```python
from build123d import *

# Parameters (mm, degrees)
F2_DEPTH = 12.5
F3_R     = 1


with BuildPart() as f1:
    # F0 (on Top) → F1 (revolve)
    with BuildSketch(Plane.XY):
        Polygon((-48.5449684441, 34.0502707809), (-50.5449684441, 34.0502707809), (-50.5449684441, 30.5502707809), (-42.7490452468, 30.5502707809), (-42.7490452468, 31.0099636614), (-39.1449684441, 31.2220901251), (-39.1449684441, 32.0502707809), (-41.1449684441, 32.7502707809), (-41.1449684441, 32.4502707809), (-48.5449684441, 32.4502707809), align=None)
        Polygon((-42.7490452468, 31.0099636614), (-42.7490452468, 30.5502707809), (-39.1449684441, 30.5502707809), (-39.1449684441, 31.2220901251), align=None)
    revolve(axis=Axis((-41.4569408685, 30.5502707809, 0), (1, 0, 0)))

    # F0 (on Top) → F2 (cut, symmetric)
    with BuildSketch(Plane.XY):
        Polygon((-42.7490452468, 31.0099636614), (-42.7490452468, 30.5502707809), (-39.1449684441, 30.5502707809), (-39.1449684441, 31.2220901251), align=None)
        Polygon((-39.1449684441, 30.5502707809), (-42.7490452468, 30.5502707809), (-42.7490452468, 30.0905779004), (-39.1449684441, 29.8784514368), align=None)
    extrude(amount=F2_DEPTH, both=True, mode=Mode.SUBTRACT)

    # F3
    f3_edges = [f1.edges().sort_by_distance(p)[0] for p in [
        (-50.544968, 27.050271, 0),
    ]]
    fillet(f3_edges, radius=F3_R)


solid = f1.part
```
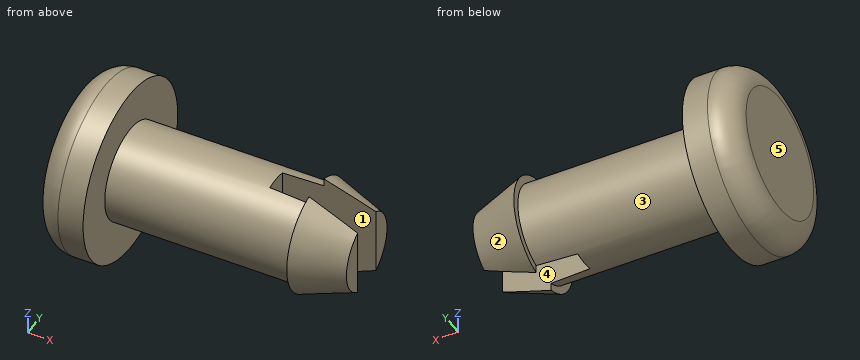
Input: part model. Units: mm. Frame: model coordinates. Face numbers are marked on the shaded views. A direction names the side the tool comes from. Give positions to 0.01 mm unless a question says otherwise; leave off trailing zeros. Loops run counter-clockwise (first coordinate to the right, second up) from the corner with the lowest first, then second, coordinate; pieces in that order, holes last. Notation, with made-up numbers: (78, -29.5) -> (102, -29.5) arc R13 ccw to (102, -12.5) -> close; hole circle Ø7 at (54.25, 37). An arc over 180 degrees is marked (long way). Use a Markdown table: item, result.
Q1. Access query for the marked faces 1 and 2. Directions: +Z, -Z, +X, -X, +Y, -Y. A direction counts if a zero-diameter tool reaches every point of the face in a straight line with its end or side. Return the directions, or none.
Entries:
| item | result |
|---|---|
| face 1 | +Z, -Z, +X |
| face 2 | +X, +Y |
Q2. Section query D-D, the plane x = -42. Return the cut outline in (y, z), plus the area to 3 significant figures.
Entries:
| item | result |
|---|---|
| outline | (30.05, -1.83) -> (30.05, 1.83) arc R1.9 ccw to start; (31.05, -1.83) arc R1.9 ccw to (31.05, 1.83) -> close |
| area | 7.56 mm² |
Q3. Ray query, probe 1 along X at (y, z) = (29.25, 2); probe 2 along Y at (x, z) = (-48, -1.25); probe 3 along Z at (x, y) = (-46, 31.75). Return the intervals inside material, ascending. Write a range as from..to.
Entries:
| item | result |
|---|---|
| probe 1 | x = -50.54..-48.54 |
| probe 2 | y = 29.12..31.98 |
| probe 3 | z = -1.47..1.47 |
Q4. Section query C-C, the plane x = -43.5. Return the cut outline in (y, z), plus the area to 3 significant figures.
Entries:
| item | result |
|---|---|
| outline | circle Ø3.8 at (30.55, 0) |
| area | 11.3 mm² |
Q5. Section query A-A, the plane z = 0. Return the cut outline in (x, y).
Entries:
| item | result |
|---|---|
| outline | (-50.54, 28.05) arc R1 ccw to (-49.54, 27.05) -> (-48.54, 27.05) -> (-48.54, 28.65) -> (-41.14, 28.65) -> (-41.14, 28.35) -> (-39.14, 29.05) -> (-39.14, 29.88) -> (-42.75, 30.09) -> (-42.75, 31.01) -> (-39.14, 31.22) -> (-39.14, 32.05) -> (-41.14, 32.75) -> (-41.14, 32.45) -> (-48.54, 32.45) -> (-48.54, 34.05) -> (-49.54, 34.05) arc R1 ccw to (-50.54, 33.05) -> close |
Q6. First-contact query: P1, Ø0.7, axis at y = 30.5, z = 0, coming from the +X side; P2, Ø3, axis at x = -41.5, y = 33, coming from the -Z side; P3, Ø1.5, axis at x = -41.5, z = 0.5, coming from the -Y side. Flat tips, straight axial feed; report the tip coordinate or a pass-through.
Entries:
| item | result |
|---|---|
| P1 | stops at x = -42.75 |
| P2 | stops at z = -1.96 |
| P3 | stops at y = 28.35 |
Q7. Pull-direction query (Y, two-part tool) for the marked faces 3, 4 and 5; classes: pulls with the +Y half, pulls with the -Y half, needs draft (parallel to the pull), parting line crosses it, or undercut.
Entries:
| item | result |
|---|---|
| face 3 | parting line crosses it |
| face 4 | undercut |
| face 5 | needs draft |
Q8. Section query B-B, the plane x = -40.75. Return the cut outline in (y, z).
Entries:
| item | result |
|---|---|
| outline | (29.97, -1.98) -> (29.97, 1.98) arc R2.06 ccw to start; (31.13, -1.98) arc R2.06 ccw to (31.13, 1.98) -> close |
